Build history of the part. All positions in model axes, mm. Round coordinates to 2 decimals unless told otherwise and drop trailing zeros. Order: outer loops, then holes, each group sorted by start corner. A loop starts at its lowest first (then second) coordinate and runs counter-clockwise, first axis right, second up. Notation, with made-up numbers: M -10,-39.75 L 30,-39.75 A20 ccw 30,-4.75 Z; hole C -23.75,84.25 d4. An arc over 180 degrees is marked long. One line per item, written item: value. Start each with the question number.
Item 1: Band-saw the part on B-B, the plane y = 2.35. Write the cut outline in (x, z) (3 decimals).
Item 2: Band-saw the part on A-A, the plane z = -7.5. Write the cut outline in (x, y) (3 decimals), then the cut area to 3 significant figures.
Item 3: Probe L1, parallel to X at y = 1.3, z = -11 (3 decimals); L2, parallel to X at y = 0.8, z = -3 (3 decimals); L3, parallel to Z at x = 57.5, y = 3. List the from-to ranges inside material, lowest first.
```python
from build123d import *

# Parameters (mm, degrees)
BOSS_EXTRUDE1_DEPTH = 3.175
SKETCH2_W           = 3.175
SKETCH2_H           = 20
CUT_EXTRUDE1_DEPTH  = 4.175
FILLET1_R           = 1


with BuildPart() as part:
    # Sketch1 → Boss-Extrude1 (new body)
    with BuildSketch(Plane(origin=(0, 0, 0), x_dir=(1, 0, 0), z_dir=(0, 1, 0))):
        with BuildLine():
            Line((5, 0), (65, 0))
            ThreePointArc((65, 0), (68.535533906, 1.464466094), (70, 5))
            Line((70, 5), (70, 35))
            ThreePointArc((70, 35), (68.535533906, 38.535533906), (65, 40))
            Line((65, 40), (5, 40))
            ThreePointArc((5, 40), (1.464466094, 38.535533906), (0, 35))
            Line((0, 35), (0, 5))
            ThreePointArc((0, 5), (1.464466094, 1.464466094), (5, 0))
        make_face()
    extrude(amount=BOSS_EXTRUDE1_DEPTH)

    # Sketch2 → Cut-Extrude1 (cut, through all)
    with BuildSketch(Plane(origin=(0, 3.175, 0), x_dir=(1, 0, 0), z_dir=(0, 1, 0))):
        with Locations((13.4125, 10)):
            Rectangle(SKETCH2_W, SKETCH2_H)
        with Locations((56.5875, 10)):
            Rectangle(SKETCH2_W, SKETCH2_H)
    extrude(amount=-CUT_EXTRUDE1_DEPTH, mode=Mode.SUBTRACT)

    # Fillet1
    fillet1_edges = [part.edges().sort_by_distance(p)[0] for p in [
        (15, 1.5875, 0),
        (58.175, 1.5875, 0),
        (55, 1.5875, 0),
        (11.825, 1.5875, 0),
    ]]
    fillet(fillet1_edges, radius=FILLET1_R)


solid = part.part
```
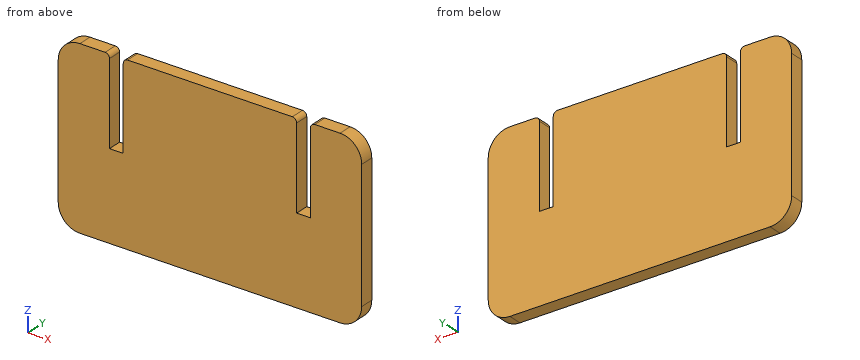
Output:
1. outline: M 0,-35 A5 ccw 5,-40 L 65,-40 A5 ccw 70,-35 L 70,-5 A5 ccw 65,0 L 59.175,0 A1 ccw 58.175,-1 L 58.175,-20 L 55,-20 L 55,-1 A1 ccw 54,0 L 16,0 A1 ccw 15,-1 L 15,-20 L 11.825,-20 L 11.825,-1 A1 ccw 10.825,0 L 5,0 A5 ccw 0,-5 Z
2. outline: M 0,0 L 11.825,0 L 11.825,3.175 L 0,3.175 Z; M 15,0 L 55,0 L 55,3.175 L 15,3.175 Z; M 58.175,0 L 70,0 L 70,3.175 L 58.175,3.175 Z
2. area: 202 mm²
3. L1: x = 0 to 11.825, 15 to 55, 58.175 to 70
3. L2: x = 0.417 to 11.825, 15 to 55, 58.175 to 69.583
3. L3: z = -40 to -20
